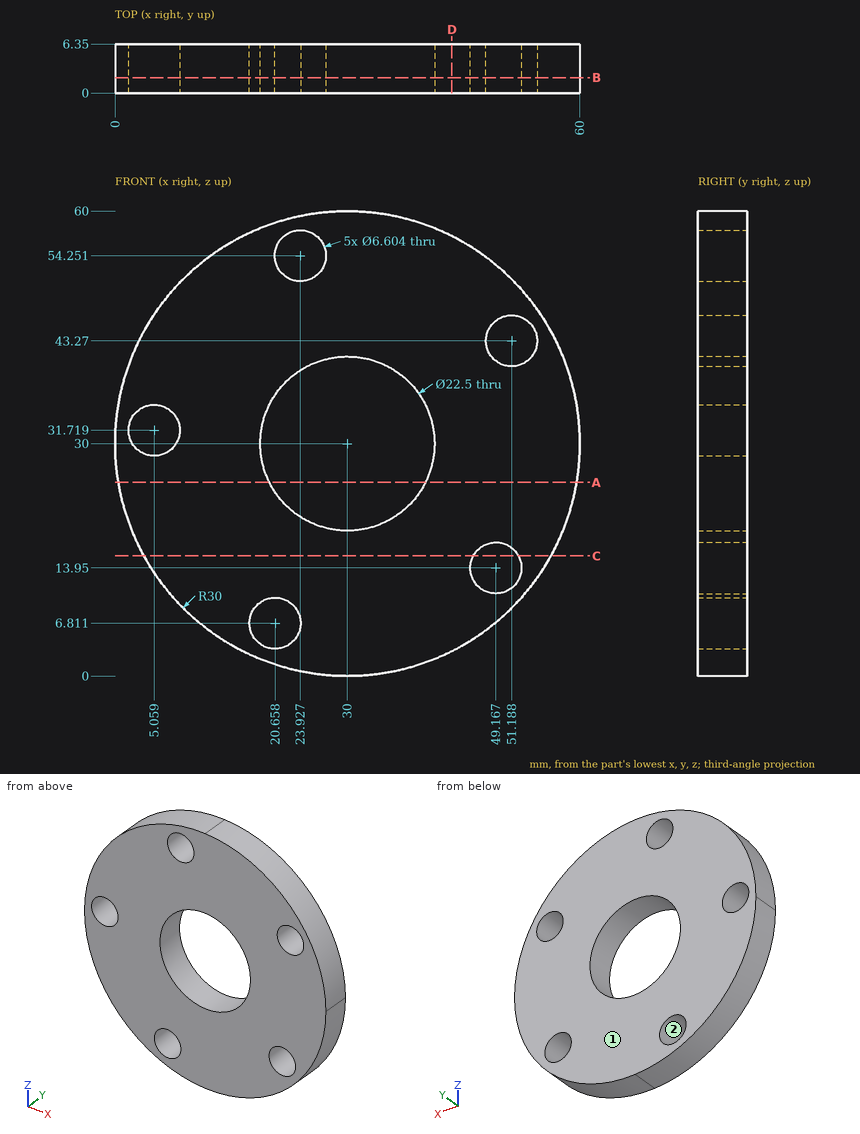
Could you check a few things on this drawing? It's one solid part, dimensions in mm from its lowest x, y, z. Give positions to 0.01 mm unless a question says otherwise; leave off trailing zeros. Order: outer loops, then holes, each group sorted by start corner. A loop starts at its lowest first (then second) coordinate and runs counter-clockwise, first axis right, second up. Notation, with made-up numbers: M -19.75,47.5 L -0.75,47.5 A34 ccw -0.75,77.5 Z; hole C 26,84 d5. An arc over 180 degrees is marked long. Use one line per item in the form item = value.
Item 1: If I drill on line 1 along Z through (x, y) = (30.5, 6) (1 decimal); line 2 along X through (y, z) = (1, 52) (1 decimal); line 3 along X through (y, z) = (2.5, 41.5) (1 decimal), over which ranges is the centre line in solid material (lowest first)? Write a range as [from, to].
Values follow:
line_1 = [0, 18.8], [41.2, 60]
line_2 = [9.6, 21.5], [26.3, 50.4]
line_3 = [2.3, 48.4], [54, 57.7]
Item 2: If we section it at D-D, the plane x = 43.5: Write out the boundary of the cut face in (y, z), and give its area (3 significant figures).
Values follow:
outline = M 0,3.21 L 6.35,3.21 L 6.35,56.79 L 0,56.79 Z
area = 340 mm^2
Item 3: If we section it at A-A, the plane z = 25: Write out the boundary of the cut face in (x, y).
Values follow:
outline = M 0.42,0 L 19.92,0 L 19.92,6.35 L 0.42,6.35 Z; M 40.08,0 L 59.58,0 L 59.58,6.35 L 40.08,6.35 Z
Item 4: Thinking about a two-plate mould opening in X: for the marked faces 1 and 2, which applies, pulls with the +X half, pulls with the -X half, needs draft (parallel to the pull), parting line crosses it, or undercut?
Values follow:
face_1 = needs draft
face_2 = undercut
Item 5: Will these pins go through, and if not, where does the flat tip stop? pin 1 Ø3 at (x, y) = (6.5, 4) entering from +Z (1 decimal); pin 2 Ø2 at (y, z) = (2, 40) entering from -X; pin 3 Ø1.5 at (y, z) = (2.5, 32) entering from +X.
Values follow:
pin_1 = 50.4
pin_2 = 1.38
pin_3 = 59.97
Item 6: If we section it at B-B, the plane y = 2: Write out the boundary of the cut face in (x, z).
Values follow:
outline = C 30,30 d60; hole C 5.06,31.72 d6.6; hole C 20.66,6.81 d6.6; hole C 30,30 d22.5; hole C 23.93,54.25 d6.6; hole C 49.17,13.95 d6.6; hole C 51.19,43.27 d6.6
Item 7: If we section it at C-C, the plane z = 15.5: Write out the boundary of the cut face in (x, y).
Values follow:
outline = M 3.74,0 L 46.25,0 L 46.25,6.35 L 3.74,6.35 Z; M 52.08,0 L 56.26,0 L 56.26,6.35 L 52.08,6.35 Z
